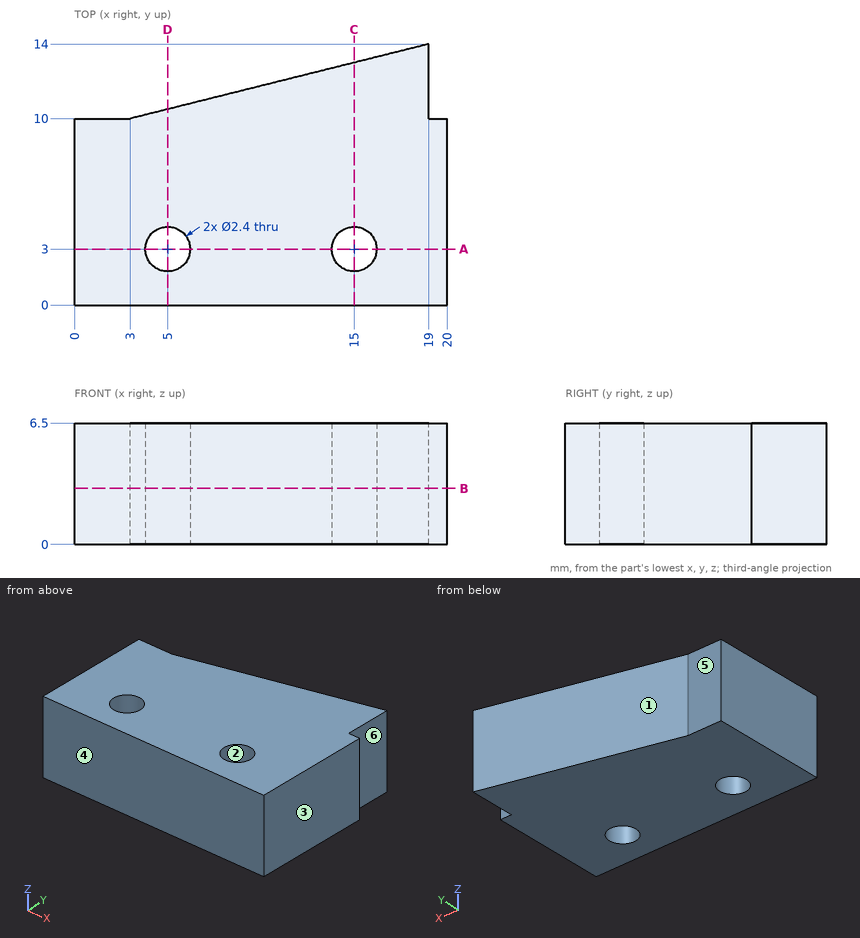
The figure shows three views and two pictorial views of one solid part (mm, origin at its lowest corner). Answer the questions. A direction names the side the tool comes from. Round coordinates to 2 decimals unless told otherwise and drop trailing zeros. Loops run counter-clockwise (first coordinate to the right, second up) from the corner with the lowest first, then second, coordinate; pieces in that order, holes last. Notation, with made-up numbers: M 61,50 L 79,50 A32 cw 79,81 Z; hole C 16,24 d6. An arc over 180 degrees is marked long. Write each question's results on one line, items separated by ' | '. Start each with the question number.
1) Find section B-B on z = 3. Write down the section's boundary in (x, y).
2) Find section C-C on x = 15. Write down the section's boundary in (y, z).
3) Find section D-D on x = 5. Write down the section's boundary in (y, z), plus the area to 4 significant figures.
4) Which of the six approach directions +Z, -Z, +X, -X, +Y, -Y give full straight-line access (tool end or side, diameter ignored) to the marked faces 4, 5 and 6?
5) Find section A-A on y = 3. Write down the section's boundary in (x, z), plus the area to 3 significant figures.
6) Straight lines are drawn through the part: probe 1 along Y at (x, z) = (14, 5.5); probe 2 along X at (y, z) = (3.5, 2.25); probe 3 along Y at (x, z) = (5, 1.75). For each, find the intervals that lie inside material, in ascending order.
7) Each of these flat-tipped pins is pushed along its axis until it touches: pin 1 (8 mm diameter, centred on x = 12, y = 4.5, fed in from -Z); pin 2 (1.2 mm diameter, centred on y = 11.5, z = 4, fed in from +X); pin 3 (3.5 mm diameter, centred on x = 1.5, z = 2.5, fed in from +Y); pin 4 (0.8 mm diameter, centred on x = 19.5, z = 4.5, fed in from +Y). Where does it stop, or does it pass through?
8) Determine the mould class of the marked faces 1, 2 and 3 for opening direction Y: pulls with the +Y half, pulls with the -Y half, needs draft (parallel to the pull), parting line crosses it, or undercut.
Final values:
1) outline: M 0,0 L 20,0 L 20,10 L 19,10 L 19,14 L 3,10 L 0,10 Z; hole C 5,3 d2.4; hole C 15,3 d2.4
2) outline: M 0,0 L 1.8,0 L 1.8,6.5 L 0,6.5 Z; M 4.2,0 L 13,0 L 13,6.5 L 4.2,6.5 Z
3) outline: M 0,0 L 1.8,0 L 1.8,6.5 L 0,6.5 Z; M 4.2,0 L 10.5,0 L 10.5,6.5 L 4.2,6.5 Z | area: 52.65 mm²
4) face 4: +Z, -Z, +X, -X, -Y | face 5: +Z, -Z, -X, +Y | face 6: +Z, -Z, +X, +Y
5) outline: M 0,0 L 3.8,0 L 3.8,6.5 L 0,6.5 Z; M 6.2,0 L 13.8,0 L 13.8,6.5 L 6.2,6.5 Z; M 16.2,0 L 20,0 L 20,6.5 L 16.2,6.5 Z | area: 98.8 mm²
6) probe 1: 0 to 2.34, 3.66 to 12.75 | probe 2: 0 to 3.91, 6.09 to 13.91, 16.09 to 20 | probe 3: 0 to 1.8, 4.2 to 10.5
7) pin 1: z = 0 | pin 2: x = 19 | pin 3: y = 10.06 | pin 4: y = 10
8) face 1: pulls with the +Y half | face 2: undercut | face 3: needs draft
